Can you work these out from the model? Positions are in its coordinate system, mm. A direction names the side the tool comes from. Give positions to 0.01 mm unless a question says otherwise; leave off trailing zeros. Write each loop counter-clockwise with the first axis right and the second up, starting at its lowest first coordinate (ties: lowest second). Pieces come first, ordered by that corner, then holes. Notation, with made-up numbers: (35.5, -25) -> (41.5, -25) arc R15 ccw to (41.5, -18) -> close; hole circle Ø3 at (19.5, -17.5). An arc over 180 degrees is marked (long way). One line per item, written item: value.
from build123d import *

# Parameters (mm, degrees)
SKETCH1_W            = 250
SKETCH1_H            = 120
BOSS_EXTRUDE1_DEPTH  = 10
M5_CLEARANCE_HOLE1_D = 5.5
CUT_EXTRUDE1_DEPTH   = 5


with BuildPart() as part:
    # Sketch1 → Boss-Extrude1 (new body)
    with BuildSketch(Plane(origin=(0, 0, 0), x_dir=(1, 0, 0), z_dir=(0, 1, 0))):
        with Locations((125, 60)):
            Rectangle(SKETCH1_W, SKETCH1_H)
    extrude(amount=BOSS_EXTRUDE1_DEPTH)

    # M5 Clearance Hole1 (through all)
    with Locations(Plane(origin=(0, 10, 0), x_dir=(1, 0, 0), z_dir=(0, 1, 0))):
        with Locations((196.625581146, 15), (207.625581146, 15), (207.625581146, 75), (196.625581146, 75)):
            m5_clearance_hole1 = Hole(M5_CLEARANCE_HOLE1_D / 2)

    # Sketch5 → Cut-Extrude1 (cut)
    with BuildSketch(Plane(origin=(0, 0, 0), x_dir=(-1, 0, 0), z_dir=(0, -1, 0))):
        with BuildLine():
            Line((-196.625581146, 8.75), (-207.625581146, 8.75))
            ThreePointArc((-207.625581146, 8.75), (-213.875581146, 15), (-207.625581146, 21.25))
            Line((-207.625581146, 21.25), (-196.625581146, 21.25))
            ThreePointArc((-196.625581146, 21.25), (-190.375581146, 15), (-196.625581146, 8.75))
        make_face()
        with BuildLine():
            Line((-196.625581146, 68.75), (-207.625581146, 68.75))
            ThreePointArc((-207.625581146, 68.75), (-213.875581146, 75), (-207.625581146, 81.25))
            Line((-207.625581146, 81.25), (-196.625581146, 81.25))
            ThreePointArc((-196.625581146, 81.25), (-190.375581146, 75), (-196.625581146, 68.75))
        make_face()
    cut_extrude1 = extrude(amount=-CUT_EXTRUDE1_DEPTH, mode=Mode.SUBTRACT)

    # Mirror1: M5 Clearance Hole1, Cut-Extrude1 across plane
    add(m5_clearance_hole1.mirror(Plane(origin=(150, 0, 0), x_dir=(0, 0, 1), z_dir=(1, 0, 0))), mode=Mode.SUBTRACT)
    add(cut_extrude1.mirror(Plane(origin=(150, 0, 0), x_dir=(0, 0, 1), z_dir=(1, 0, 0))), mode=Mode.SUBTRACT)


solid = part.part
1) For faces 1 (the face through (190.377, 2.465, -15.137)), 2 (the face through (199.373, 7.465, -75.121)), which set-ups out of +Z, -Z, +X, -X, +Y, -Y let a thin tool reach every point of the face, with its end or its side?
Answer list:
face 1: -Y
face 2: +Y, -Y
2) Will these pins go through, and if not, where does the flat tip stop? pin 1 (6 mm diameter, centred on x = 96, z = -77, fed in from -Y); pin 2 (5 mm diameter, centred on x = 196.63, z = -75, fed in from +Y) (3 decimals).
Answer list:
pin 1: stops at y = 5
pin 2: passes through
3) If we section it at B-B (y = 3.5): Write out the boundary of the cut face in (x, z), and give its area (3 significant figures).
Answer list:
outline: (0, -120) -> (250, -120) -> (250, 0) -> (0, 0) -> close; hole (92.37, -81.25) -> (103.37, -81.25) arc R6.25 ccw to (103.37, -68.75) -> (92.37, -68.75) arc R6.25 ccw to start; hole (92.37, -21.25) -> (103.37, -21.25) arc R6.25 ccw to (103.37, -8.75) -> (92.37, -8.75) arc R6.25 ccw to start; hole (196.63, -81.25) -> (207.63, -81.25) arc R6.25 ccw to (207.63, -68.75) -> (196.63, -68.75) arc R6.25 ccw to start; hole (196.63, -21.25) -> (207.63, -21.25) arc R6.25 ccw to (207.63, -8.75) -> (196.63, -8.75) arc R6.25 ccw to start
area: 29,000 mm^2
4) If we section it at A-A (z = -15): Write out the boundary of the cut face in (x, y), and give its area (4 significant figures).
Answer list:
outline: (0, 0) -> (86.12, 0) -> (86.12, 5) -> (89.62, 5) -> (89.62, 10) -> (0, 10) -> close; (95.12, 5) -> (100.62, 5) -> (100.62, 10) -> (95.12, 10) -> close; (106.12, 5) -> (109.62, 5) -> (109.62, 0) -> (190.38, 0) -> (190.38, 5) -> (193.88, 5) -> (193.88, 10) -> (106.12, 10) -> close; (199.38, 5) -> (204.88, 5) -> (204.88, 10) -> (199.38, 10) -> close; (210.38, 5) -> (213.88, 5) -> (213.88, 0) -> (250, 0) -> (250, 10) -> (210.38, 10) -> close
area: 2,155 mm^2
5) I need wall thicknesses on L1, parallel to X at y = 2, z = -72; L2, parallel to Z at x = 88.5, y = 4.5. Which ranges of each line are inside material? Lowest first, please.
Answer list:
L1: x = 0 to 86.89, 108.86 to 191.14, 213.11 to 250
L2: z = -120 to -79.9, -70.1 to -19.9, -10.1 to 0
6) We'd pull the mould along Z, two halves only. Please class faces 3 (the face through (250, 5, -59)), 4 (the face through (109.623, 2.465, -75.137)): released by +Z, released by -Z, zero draft, split by the parting line, or undercut.
Answer list:
face 3: zero draft
face 4: undercut
